Build history of the part. All positions in model axes, mm. Face numbers are marked on the shaded views. A direction names the side the tool comes from. Round coordinates to 2 decimals unless told otherwise and drop trailing zeros. Order: outer loops, then holes, each group sorted by start corner. A loop starts at its lowest first (then second) coordinate and runs counter-clockwise, first axis right, second up. Notation, with made-up numbers: (17, 1.5) -> (23, 1.5) arc R11 cw to (23, 20.5) -> close; hole circle Ø10 at (80.5, 75). An arc over 180 degrees is marked (long way). Use a Markdown table: item, result. Add a question column.
Item 1: Slice it at B-B, the plane x = 8. Give the cut face in (y, z), plus the area to 3 significant figures.
Item 2: Slice it at C-C, the plane y = -47. Give the cut face in (x, z).
Item 3: Slice it at A-A, the plane z = -24. Give the cut face in (x, y), plus the area to 3 significant figures.
Item 4: Probe L1, parallel to Y at x = -5, z = -35.5; L2, parallel to Z at x = -10, y = -23; L3, parallel to Z at x = 23.5, y = -27.5. List the from-to ranges inside material, lowest first.
Item 5: Pin check, flat tips, straight feed: pin 1 (2 mm diameter, centred on x = -11, z = 8, fed in from -Y); pin 2 (1 mm diameter, centred on y = -11, z = 21, fed in from +X); pin 3 (5 mm diameter, centred on x = -12.5, y = -85.5, fed in from +Z). Stop position of each tip, or through.
Item 6: Two-plate mould, pull along Z, no slides. Class the marked faces 3, 4 and 5: released by +Z, released by -Z, zero draft, split by the parting line, or undercut.
Item 7: Slice it at D-D, the plane z = 18.5. Give the cut face in (x, y).
Item 8: 3-axis set-ups, long thin cutter, end or side, ignore diameter. For the marked faces 1 and 2: which of +Z, -Z, +X, -X, +Y, -Y reach the whole face in a straight line?
from build123d import *

# Parameters (mm, degrees)
PAD_DEPTH       = 90
POCKET_DEPTH    = 10
SKETCH002_W     = 15.977638
SKETCH002_H     = 29.995947
POCKET001_DEPTH = 10
SKETCH003_W     = 7.803505
SKETCH003_H     = 10.033076
POCKET002_DEPTH = 10
SKETCH004_W     = 7.580546
SKETCH004_H     = 9.884439
SKETCH004_W_2   = 7.506227
SKETCH004_H_2   = 9.364204
SKETCH004_W_3   = 7.952141
SKETCH004_H_3   = 8.992611
POCKET003_DEPTH = 10


with BuildPart() as part:
    # Sketch → Pad (new body)
    with BuildSketch(Plane.XZ):
        Polygon((0, 30.192584), (-30.283876, 0), (-30.283876, -40.257482), (29.976444, -40.257482), (29.976444, 0), align=None)
    extrude(amount=PAD_DEPTH)

    # Sketch001 (on Face7 of Pad) → Pocket (cut)
    with BuildSketch(Plane.XZ.offset(90)):
        Polygon((0, 25.187876), (25.062579, 0), (-24.79101, 0), align=None)
    extrude(amount=-POCKET_DEPTH, mode=Mode.SUBTRACT)

    # Sketch002 (on Face5 of Pocket) → Pocket001 (cut)
    with BuildSketch(Plane.XZ.offset(90)):
        with Locations((-12.082496, -25.124813)):
            Rectangle(SKETCH002_W, SKETCH002_H)
    extrude(amount=-POCKET001_DEPTH, mode=Mode.SUBTRACT)

    # Sketch003 (on Face5 of Pocket001) → Pocket002 (cut)
    with BuildSketch(Plane.XZ.offset(90)):
        with Locations((8.075235, -15.109341)):
            Rectangle(SKETCH003_W, SKETCH003_H)
    extrude(amount=-POCKET002_DEPTH, mode=Mode.SUBTRACT)

    # Sketch004 (on Face5 of Pocket002) → Pocket003 (cut)
    with BuildSketch(Plane.XZ.offset(90)):
        with Locations((17.978553, -15.130553)):
            Rectangle(SKETCH004_W, SKETCH004_H)
        with Locations((7.833998, -26.538534)):
            Rectangle(SKETCH004_W_2, SKETCH004_H_2)
        with Locations((18.015712, -26.798651)):
            Rectangle(SKETCH004_W_3, SKETCH004_H_3)
    extrude(amount=-POCKET003_DEPTH, mode=Mode.SUBTRACT)


solid = part.part
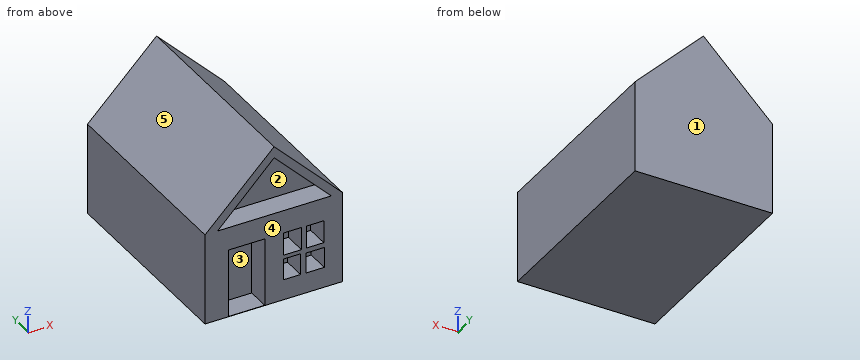
Check sheet entries:
| question | item | result |
|---|---|---|
| 1 | outline | (-90, -40.26) -> (0, -40.26) -> (0, 22.13) -> (-90, 22.13) -> (-90, 17.15) -> (-80, 17.15) -> (-80, 0) -> (-90, 0) -> (-90, -10.09) -> (-80, -10.09) -> (-80, -20.13) -> (-90, -20.13) -> (-90, -21.86) -> (-80, -21.86) -> (-80, -31.22) -> (-90, -31.22) -> close |
| 1 | area | 5,250 mm2 |
| 2 | outline | (-30.28, -40.26) -> (29.98, -40.26) -> (29.98, 0) -> (0, 30.19) -> (-30.28, 0) -> close |
| 3 | outline | (-30.28, -90) -> (-20.07, -90) -> (-20.07, -80) -> (-4.09, -80) -> (-4.09, -90) -> (4.08, -90) -> (4.08, -80) -> (11.59, -80) -> (11.59, -90) -> (14.04, -90) -> (14.04, -80) -> (21.99, -80) -> (21.99, -90) -> (29.98, -90) -> (29.98, 0) -> (-30.28, 0) -> close |
| 3 | area | 5,110 mm2 |
| 4 | L1 | -80 to 0 |
| 4 | L2 | -40.26 to 20.22 |
| 4 | L3 | -40.26 to 6.52 |
| 5 | pin 1 | y = -80 |
| 5 | pin 2 | x = 9.62 |
| 5 | pin 3 | z = 20.22 |
| 6 | face 3 | undercut |
| 6 | face 4 | zero draft |
| 6 | face 5 | released by +Z |
| 7 | outline | (-11.73, -90) -> (-6.58, -90) -> (-6.58, -80) -> (6.65, -80) -> (6.65, -90) -> (11.61, -90) -> (11.61, 0) -> (-11.73, 0) -> close |
| 8 | face 1 | +Z, -Z, +X, -X, +Y |
| 8 | face 2 | -Y |
